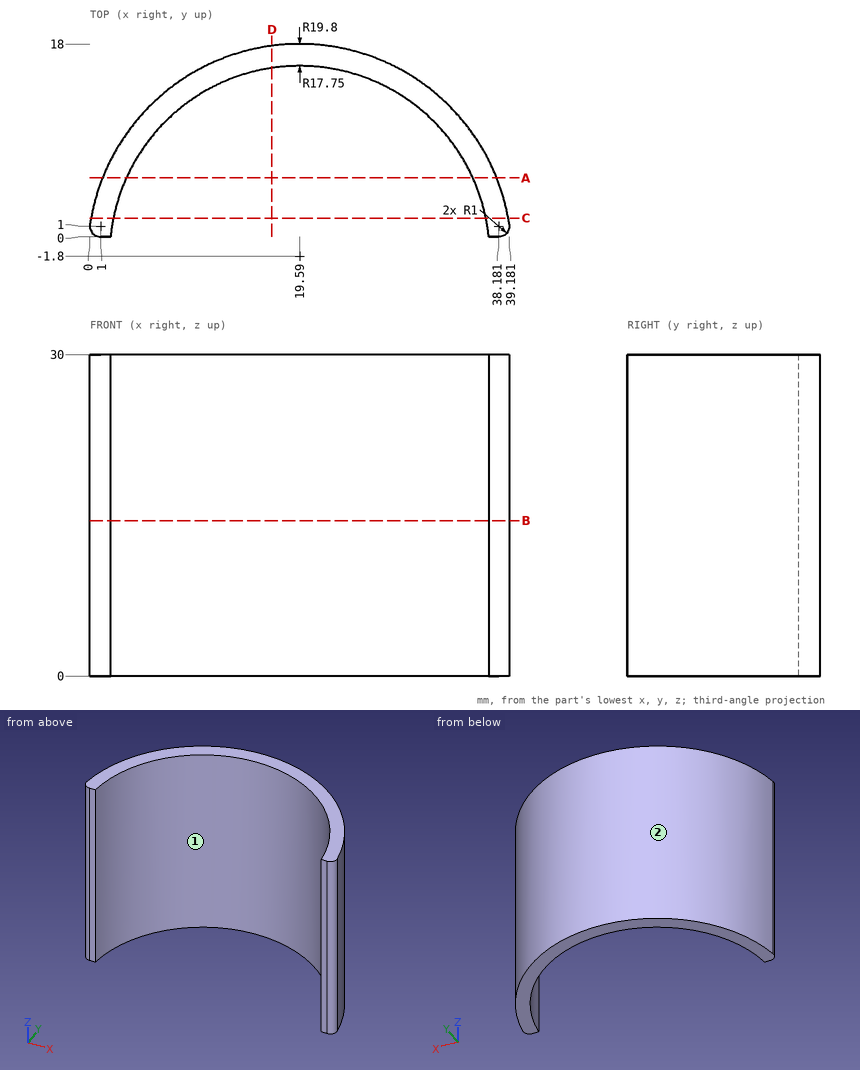
The figure shows three views and two pictorial views of one solid part (mm, origin at its lowest corner). Answer the questions. Coordinates: 2 decimals unless noted, no trailing zeros. Write each loop counter-clockwise with the first axis right and the second up, starting at its lowest first coordinate (ties: lowest second). Pieces come first, ordered by that corner, then holes. Notation, with made-up numbers: M 62,51 L 107,51 A25 cw 107,71 Z; hole C 36.5,17.25 d6. An arc over 180 degrees is marked long. Answer as CSV lines item,"result". Start each with the question number.
Item 1: Section A-A on y = 5.5 is taken. Write down the section's boundary in (x, z) (1 decimal).
Item 2: Consider L1, parallel to Y at x = 19.5, z = 10.75; L2, parallel to X at y = 2.75, z = 12.25; L3, parallel to X at y = 3.25, z = 26.5 (1 decimal). Determine where each line is inside the solid, lowest interval first.
Item 3: Flat-ended cylindrical pins translate along their axes: P1, Ø2, axis at y = 3.5, z = 19.5, coming from the +X side; P2, Ø3, axis at x = 30, y = 14, coming from the -Z side; P3, Ø8, axis at x = 18.5, z = 26, coming from the -Y side (1 decimal); P4, Ø10, axis at x = 13, z = 15.5, coming from the -Y side. Find the tip coordinate at first contact, or state that the pin passes through.
Item 4: Section D-D on x = 17 is taken. Write down the section's boundary in (y, z).
Item 5: Determine the mould class of the marked faces 1 and 2 for opening direction X: released by +X, released by -X, zero draft, split by the parting line, or undercut.
Item 6: Section C-C on y = 1.75 is taken. Write down the section's boundary in (x, z), and give its area (3 significant figures).
Item 7: Section B-B on z = 14.5 is taken. Write down the section's boundary in (x, y), and give its area (3 significant figures).
Checks:
1,outline,"M 1.2,0 L 3.4,0 L 3.4,30 L 1.2,30 Z; M 35.8,0 L 38,0 L 38,30 L 35.8,30 Z"
2,L1,"y = 15.95 to 18"
2,L2,"x = 0.32 to 2.43, 36.75 to 38.86"
2,L3,"x = 0.4 to 2.6, 36.6 to 38.7"
3,P1,"stops at x = 38.92"
3,P2,"stops at z = 0"
3,P3,"stops at y = 15.2"
3,P4,"stops at y = 11.64"
4,outline,"M 15.76,0 L 17.83,0 L 17.83,30 L 15.76,30 Z"
5,face 1,"undercut"
5,face 2,"split by the parting line"
6,outline,"M 0.11,0 L 2.2,0 L 2.2,30 L 0.11,30 Z; M 36.98,0 L 39.07,0 L 39.07,30 L 36.98,30 Z"
6,area,"125 mm²"
7,outline,"M 0.01,1.15 A1 ccw 1,0 L 1.93,0 A17.75 cw 37.25,0 L 38.18,0 A1 ccw 39.17,1.15 A19.8 ccw Z"
7,area,"113 mm²"
